Can you work these out from the drawing? Everything is in mm from the part's minimum corner. Round coordinates to 2 decimals unless told otherwise and drop trailing zeros. Order: outer loops, then holes, each group sorted by start corner. A loop starts at its lowest first (then second) coordinate and runs counter-clockwise, first axis right, second up. Notation, with made-up numbers: M -13.5,12.5 L 15.5,12.5 A29 cw 15.5,45.5 Z; hole C -21.5,30 d11. An arc over 180 degrees is marked long. Answer as a JSON object with one key per item and string values. Group by question number.
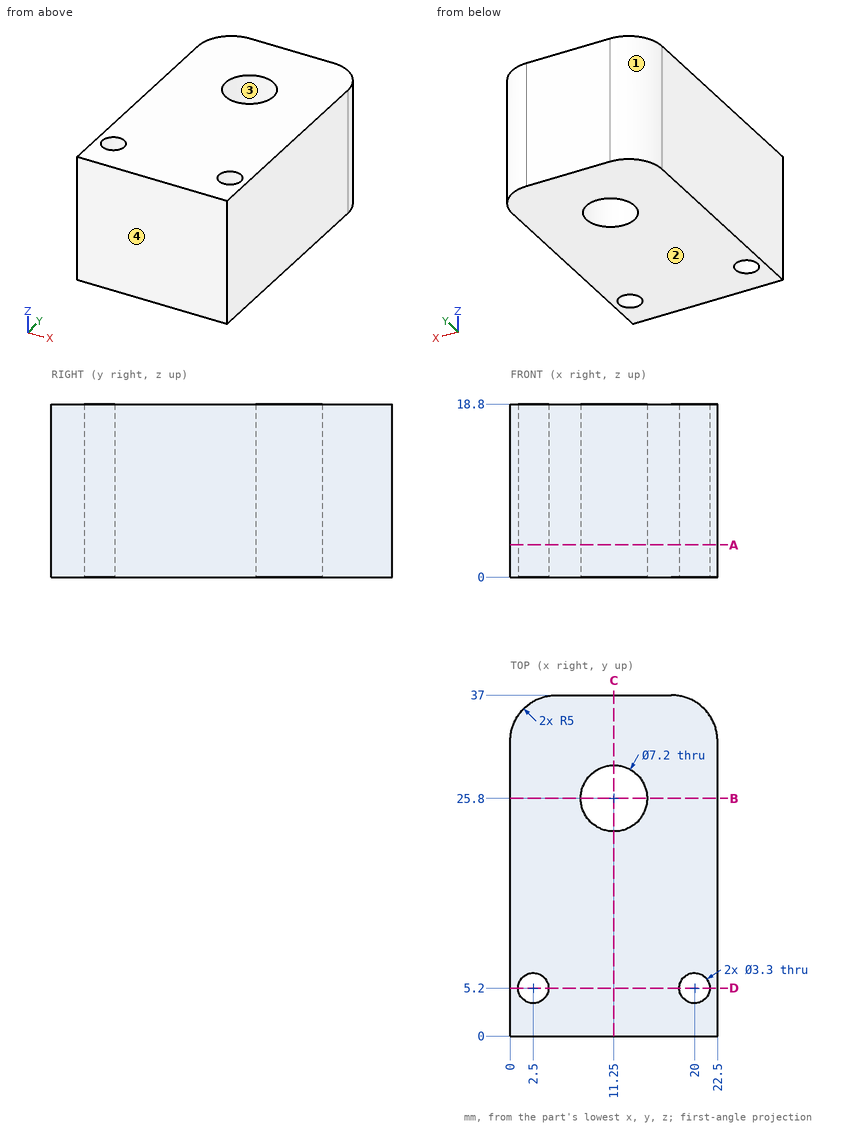
Item 1: Suppose I cut it at A-A, the plane z = 3.5. Write out the boundary of the cut face in (x, y), and give its area (3 significant figures).
Item 2: Suppose I cut it at C-C, the plane x = 11.25. Write out the boundary of the cut face in (y, z), and give its area (3 significant figures).
Item 3: I'm going to push a flat-ended pin straight in: pin 1 Ø6 at (x, y) = (14.5, 15.5) entering from -Z. Where does the tip first touch, or does it pass through?
Item 4: Suppose I cut it at B-B, the plane y = 25.8. Write out the boundary of the cut face in (x, z).
Item 5: If we mould it in two halves opening along Y, with no side actions, what happens to the marked faces 1, 2, 3 and 4? For each: +Y half, -Y half, draft (parallel to the pull), parting line (faces both ways), or undercut.
Item 6: Suppose I cut it at D-D, the plane y = 5.2. Write out the boundary of the cut face in (x, z), and give its area (3 significant figures).
Item 7: I need wall thicknesses on line 1 (Y direction, x = 11.25, z = 7); line 2 (X direction, y = 4, z = 5); line 3 (Y direction, x = 20, z = 6). Which ranges of each line are inside material? Lowest first, please.
Computed:
{
 "1": {"outline": "M 0,0 L 22.5,0 L 22.5,32 A5 ccw 17.5,37 L 5,37 A5 ccw 0,32 Z; hole C 2.5,5.2 d3.3; hole C 11.25,25.8 d7.2; hole C 20,5.2 d3.3", "area": "764 mm^2"},
 "2": {"outline": "M 0,0 L 22.2,0 L 22.2,18.8 L 0,18.8 Z; M 29.4,0 L 37,0 L 37,18.8 L 29.4,18.8 Z", "area": "560 mm^2"},
 "3": {"pin 1": "stops at z = 0"},
 "4": {"outline": "M 0,0 L 7.65,0 L 7.65,18.8 L 0,18.8 Z; M 14.85,0 L 22.5,0 L 22.5,18.8 L 14.85,18.8 Z"},
 "5": {"face 1": "+Y half", "face 2": "draft", "face 3": "undercut", "face 4": "-Y half"},
 "6": {"outline": "M 0,0 L 0.85,0 L 0.85,18.8 L 0,18.8 Z; M 4.15,0 L 18.35,0 L 18.35,18.8 L 4.15,18.8 Z; M 21.65,0 L 22.5,0 L 22.5,18.8 L 21.65,18.8 Z", "area": "299 mm^2"},
 "7": {"line 1": "y = 0 to 22.2, 29.4 to 37", "line 2": "x = 0 to 1.37, 3.63 to 18.87, 21.13 to 22.5", "line 3": "y = 0 to 3.55, 6.85 to 36.33"}
}
